Could you check a few things on this drawing? It's one solid part, dimensions in mm from its lowest x, y, z. A direction names the side the tool comes from. Give positions to 0.01 mm unless a question says otherwise; leave off trailing zeros. Loops run counter-clockwise (first coordinate to the right, second up) from the corner with the lowest first, then second, coordinate; pieces in that order, holes last. Notation, with made-up numbers: (4.5, 9) - (58.5, 9) arc R12 cw to (58.5, 25) - close; hole circle Ø8 at (-31.75, 43). An arc over 180 degrees is marked (long way). Put each result on its own line as item: value. Start each with the question number.
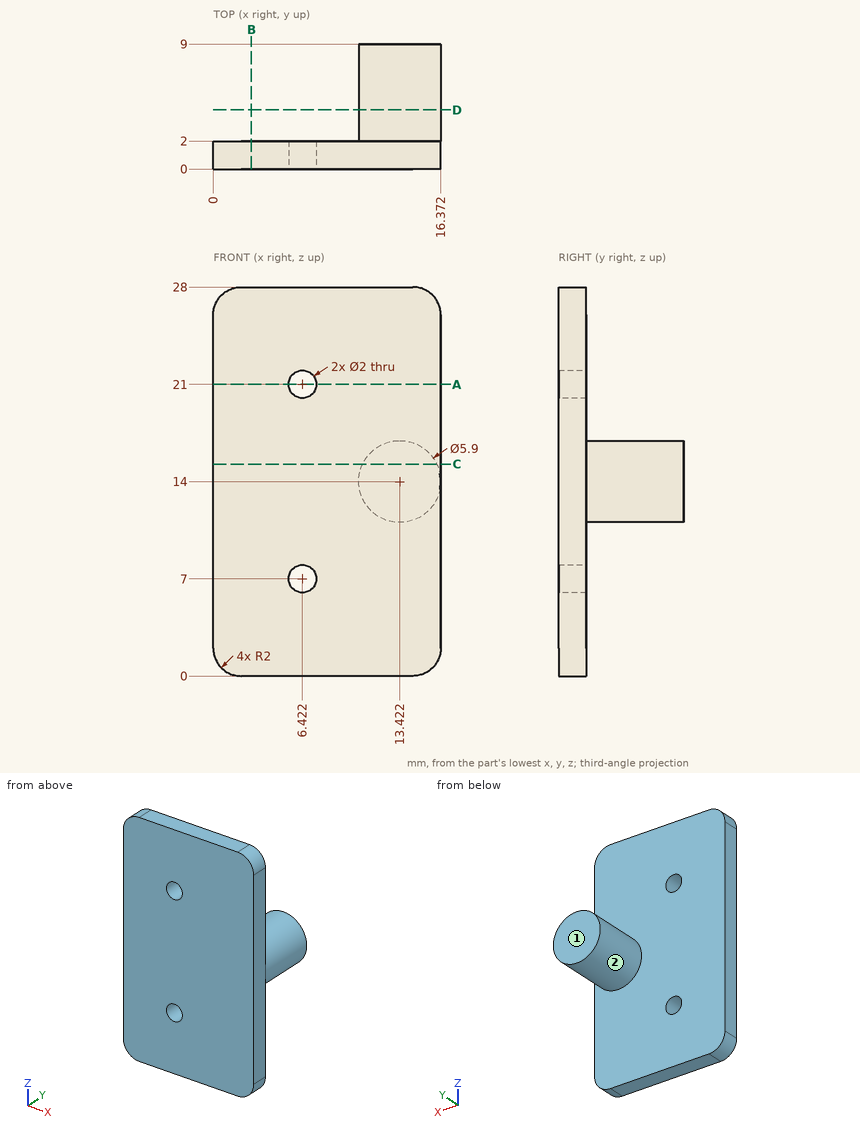
1) Suppose I cut it at D-D on y = 4.25. Please give me the cut outline in (x, z), plus the area to 3 significant figures.
2) Suppose I cut it at B-B on x = 2.75. Please give me the cut outline in (y, z), plus the area to 3 significant figures.
3) I'm going to push flat-ended pins straight in: P1, Ø1.2, axis at x = 6.42, z = 21, coming from the -Y side; P2, Ø1.5, axis at y = 7, z = 14.5, coming from the -X side. Where does each tip first touch, or does it pass through?
4) Suppose I cut it at C-C on z = 15.25. Please give me the cut outline in (x, y).
5) Suppose I cut it at A-A on z = 21. Please give me the cut outline in (x, y).
6) Which directions (+Z, -Z, +X, -X, +Y, -Y) give clear straight access to the entire face, cutting with the end or side of a thin tool? Please do the marked faces 1 and 2.
7) I need wall thicknesses on line 1 (X direction, y = 1.45, z = 21); line 2 (Y direction, x = 8, z = 6.75); line 3 (Z direction, x = 14.25, y = 8.5). Which ranges of each line are inside material? Lowest first, please.
Ans:
1. outline: circle Ø5.9 at (13.42, 14)
1. area: 27.3 mm²
2. outline: (0, 0) - (2, 0) - (2, 28) - (0, 28) - close
2. area: 56.0 mm²
3. P1: passes through
3. P2: stops at x = 10.47
4. outline: (0, 0) - (16.37, 0) - (16.37, 2) - (16.09, 2) - (16.09, 9) - (10.75, 9) - (10.75, 2) - (0, 2) - close
5. outline: (0, 0) - (5.42, 0) - (5.42, 2) - (0, 2) - close; (7.42, 0) - (16.37, 0) - (16.37, 2) - (7.42, 2) - close
6. face 1: +Z, -Z, +X, -X, +Y
6. face 2: +Y
7. line 1: x = 0 to 5.42, 7.42 to 16.37
7. line 2: y = 0 to 2
7. line 3: z = 11.17 to 16.83
